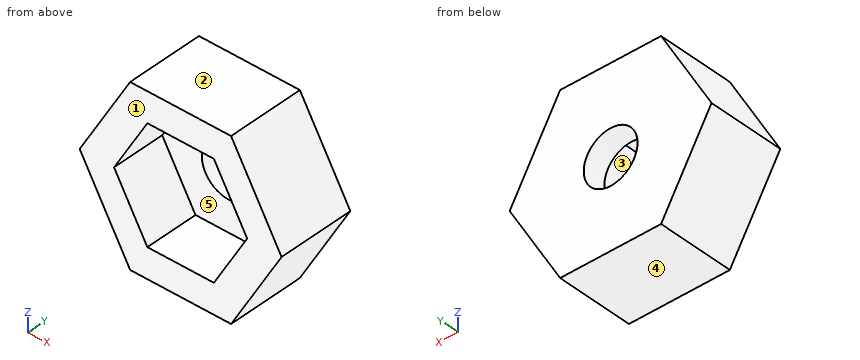
```python
from build123d import *

# Parameters (mm, degrees)
F1_DEPTH = 5.08
F3_DEPTH = 3.556
F4_R     = 1.778
F5_DEPTH = 5.081


with BuildPart() as f1:
    # F0 (on Front) → F1 (new body)
    with BuildSketch(Plane.XZ):
        Polygon((3.336219, 5.7785), (-3.336219, 5.7785), (-6.672437, 0), (-3.336219, -5.7785), (3.336219, -5.7785), (6.672437, 0), align=None)
    extrude(amount=F1_DEPTH)

    # F2 (on face) → F3 (cut)
    with BuildSketch(Plane.XZ.offset(5.08)):
        Polygon((-2.199705, -3.81), (2.199705, -3.81), (4.399409, 0), (2.199705, 3.81), (-2.199705, 3.81), (-4.399409, 0), align=None)
    extrude(amount=-F3_DEPTH, mode=Mode.SUBTRACT)

    # F4 (on face) → F5 (cut, through all)
    with BuildSketch(Plane(origin=(0, 0, 0), x_dir=(-1, 0, 0), z_dir=(0, 1, 0))):
        Circle(F4_R)
    extrude(amount=-F5_DEPTH, mode=Mode.SUBTRACT)


solid = f1.part
```
Check sheet for the modelled part. Datum: model origin and axes. Units: mm. Face numbers are marked on the shaded views. A direction names the side the tool comes from. Round coordinates to 2 decimals unless told otherwise and drop trailing zeros. Write each loop counter-clockwise with the first axis right and the second up, starting at its lowest first coordinate (ties: lowest second). Pieces come first, ordered by that corner, then holes. Notation, with made-up numbers: (36, -27) -> (43, -27) arc R23 ccw to (43, 10) -> close; hole circle Ø10 at (-19.75, 56). An arc over 180 degrees is marked (long way). Put each result on its own line as item: value.
(1) Sectioned sample at D-D (y = -4). Enter the section's corners in (x, z), plus the area to 3 significant figures.
Values found:
outline: (-6.67, 0) -> (-3.34, -5.78) -> (3.34, -5.78) -> (6.67, 0) -> (3.34, 5.78) -> (-3.34, 5.78) -> close; hole (-4.4, 0) -> (-2.2, -3.81) -> (2.2, -3.81) -> (4.4, 0) -> (2.2, 3.81) -> (-2.2, 3.81) -> close
area: 65.4 mm^2
(2) Sectioned sample at A-A (x = 0). Enter the section's corners in (y, z).
Values found:
outline: (-5.08, -5.78) -> (0, -5.78) -> (0, -1.78) -> (-1.52, -1.78) -> (-1.52, -3.81) -> (-5.08, -3.81) -> close; (-5.08, 3.81) -> (-1.52, 3.81) -> (-1.52, 1.78) -> (0, 1.78) -> (0, 5.78) -> (-5.08, 5.78) -> close
(3) Go/stop test with flat-tipped pins: pin 1 Ø1 at (y, z) = (-3, -1.5) entering from +X; pin 2 Ø4 at (x, z) = (-1.5, -2) entering from -Y; pin 3 Ø1.5 at (y, z) = (-2.5, -2) entering from -X; pin 4 Ø1.5 at (y, z) = (-4.5, -0.5) entering from +X. Record where each tip stops, or that it passes through.
Values found:
pin 1: stops at x = 6.1
pin 2: stops at y = -5.08
pin 3: stops at x = -5.95
pin 4: stops at x = 6.67
(4) Tool access check on the marked faces 4 and 5. Record the directions out of +Z, -Z, +X, -X, +Y, -Y that give a thin tool (end or side, any length) a straight path to the whole face; none if there is none.
Values found:
face 4: -Z, +X, -X, +Y, -Y
face 5: -Y
(5) Mould release check, pull along Z, two halves, no side actions. Record for the marked faces 1, 2 and 3: released by +Z, released by -Z, zero draft, split by the parting line, or undercut.
Values found:
face 1: zero draft
face 2: released by +Z
face 3: undercut
(6) Sectioned sample at B-B (y = -0.35). Enter the section's corners in (x, z).
Values found:
outline: (-6.67, 0) -> (-3.34, -5.78) -> (3.34, -5.78) -> (6.67, 0) -> (3.34, 5.78) -> (-3.34, 5.78) -> close; hole circle Ø3.56 at (0, 0)
(7) Sectioned sample at C-C (z = -1). Enter the section's corners in (x, y), plus the area to 3 significant figures.
Values found:
outline: (-6.1, -5.08) -> (-3.82, -5.08) -> (-3.82, -1.52) -> (-1.47, -1.52) -> (-1.47, 0) -> (-6.1, 0) -> close; (1.47, -1.52) -> (3.82, -1.52) -> (3.82, -5.08) -> (6.1, -5.08) -> (6.1, 0) -> (1.47, 0) -> close
area: 30.3 mm^2
(8) Material ranges on line 1 (Z direction, x = 0, y = -0.5); line 2 (Z direction, x = 1, y = -4.25); line 3 (Y direction, x = -2.5, z = -1.5), recorded low to high.
Values found:
line 1: z = -5.78 to -1.78, 1.78 to 5.78
line 2: z = -5.78 to -3.81, 3.81 to 5.78
line 3: y = -1.52 to 0
